Could you check a few things on this drawing? It's one solid part, dimensions in mm from its lowest x, y, z. Coordinates: 2 decimals unless noted, no trailing zeros. Order: outer loops, then holes, each group sorted by start corner. A loop starts at its lowest first (then second) coordinate and runs counter-clockwise, first axis right, second up. Notation, with made-up numbers: M -34,19 L 8,19 A19 ccw 8,43 Z; hole C -19,38 d4. An arc over 180 degrees is marked long. Answer as CSV lines item,"result". Start each with the question number.
1. I need wall thicknesses on line 1 along X through (y, z) = (2.25, 35); line 2 along Z through (x, y) = (160.5, 1.8). Which ranges of each line are inside material? Lowest first, please. Write a range as from..to.
2. If we section it at A-A (z = 69): List the corners of the cut face in (x, y) for me, plus the area to 3 significant figures.
3. If we section it at B-B (x = 138.5): List the corners of the cut face in (y, z) for me.
4. If we section it at C-C (y = 0.95): List the corners of the cut face in (x, z) for me.
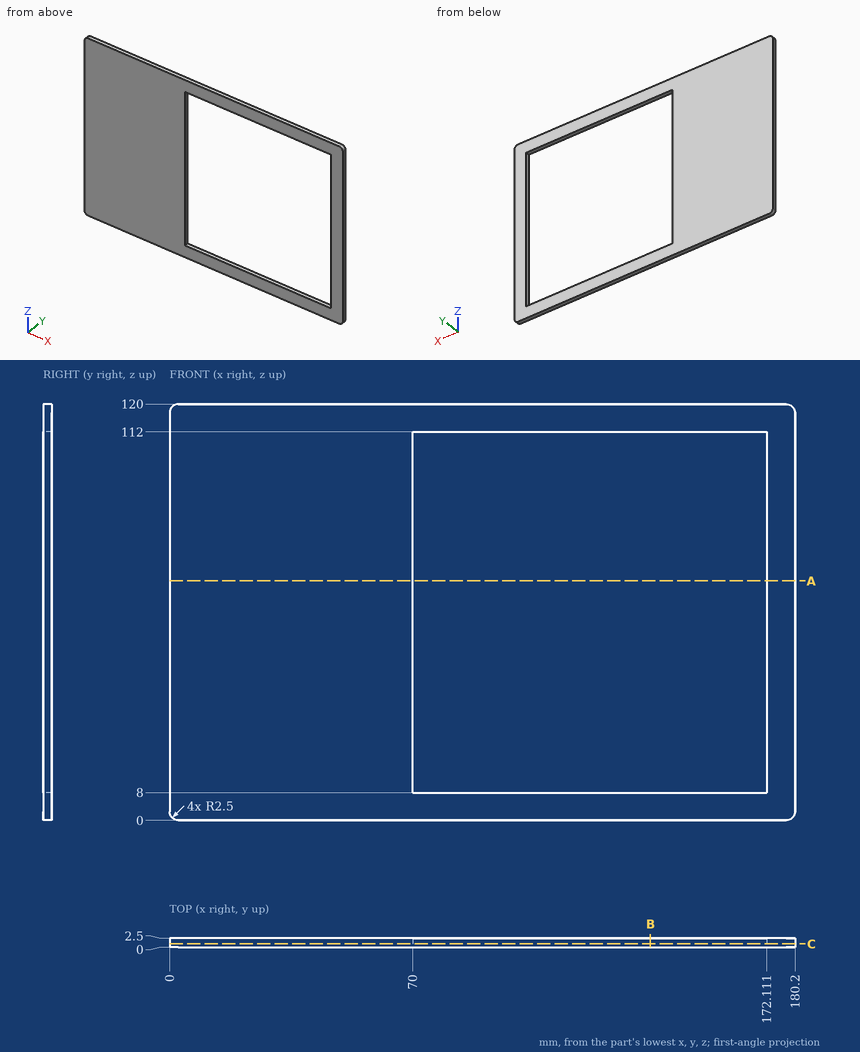
Solved:
1,line 1,"0..70, 172.11..180.2"
1,line 2,"0..8, 112..120"
2,outline,"M 0,0 L 70,0 L 70,2.5 L 0,2.5 Z; M 172.11,0 L 180.2,0 L 180.2,2.5 L 172.11,2.5 Z"
2,area,"195 mm²"
3,outline,"M 0,0 L 2.5,0 L 2.5,8 L 0,8 Z; M 0,112 L 2.5,112 L 2.5,120 L 0,120 Z"
4,outline,"M 0,2.5 A2.5 ccw 2.5,0 L 177.7,0 A2.5 ccw 180.2,2.5 L 180.2,117.5 A2.5 ccw 177.7,120 L 2.5,120 A2.5 ccw 0,117.5 Z; hole M 70,8 L 172.11,8 L 172.11,112 L 70,112 Z"
